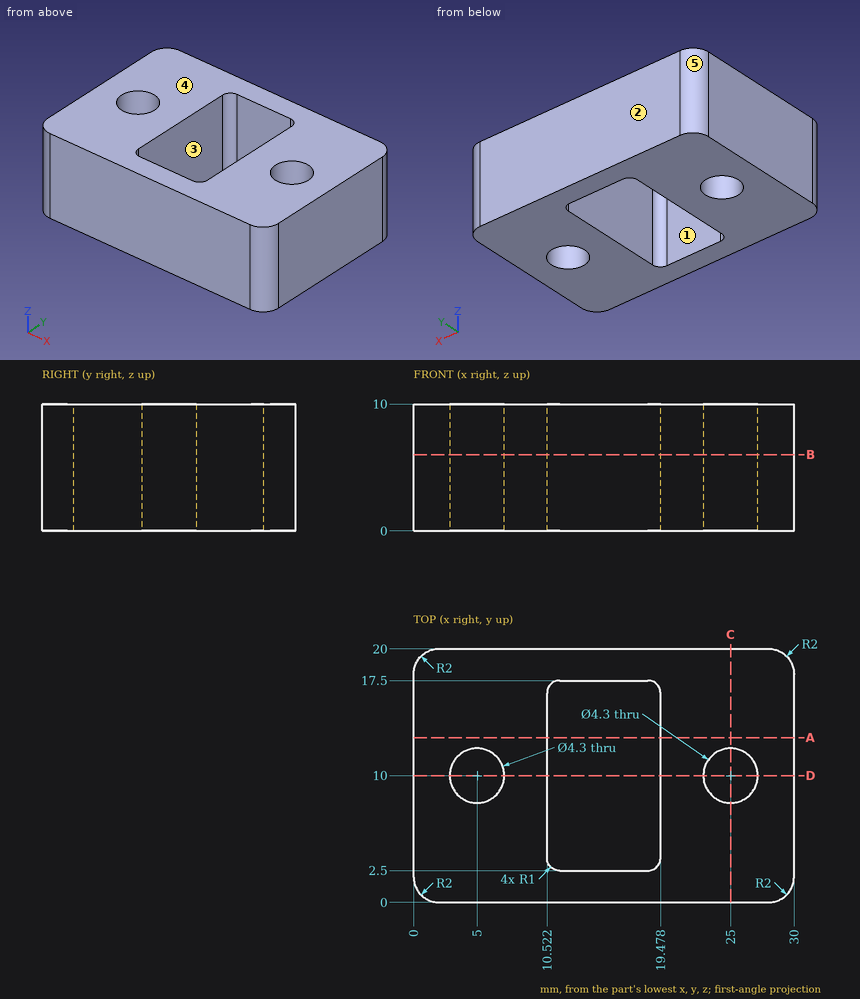
Part print with two shaded views. Sizes in mm from the minimum x, y, z corner. A direction names the side the tool comes from. Give positions to 0.01 mm unless a question says otherwise; leave off trailing zeros. Order: outer loops, then holes, each group sorted by start corner. A loop starts at its lowest first (then second) coordinate and runs counter-clockwise, first axis right, second up.
(1) Mould opens along Y. For the marked faces 3, 4 and 5 say: released by +Y, released by -Y, zero draft, split by the parting line, or undercut.
(2) Saw through at C-C, the plane x = 25. Give the cut face in (y, z), then the cut area to 3 significant figures.
(3) Saw through at A-A, the plane y = 13. Give the cut face in (x, z).
(4) Drill centre lines: L1, parallel to Y at x = 16.5, z = 4; L2, parallel to X at y = 14.25, z = 9.25; L3, parallel to Y at x = 25, z = 6.75. Where is each one in solid material? Low to high.
(5) Saw through at B-B, the plane z = 6. Give the cut face in (x, y).
(6) Tool access for the marked faces 1 and 2: list every direction of +Z, -Z, +X, -X, +Y, -Y with a clear straight run to the whole face (end or side of a thin tool).
(7) Saw through at D-D, the plane y = 10. Give the cut face in (x, z), then the cut area to 3 significant figures.
Results found:
1. face 3: undercut
1. face 4: zero draft
1. face 5: released by +Y
2. outline: (0, 0) - (7.85, 0) - (7.85, 10) - (0, 10) - close; (12.15, 0) - (20, 0) - (20, 10) - (12.15, 10) - close
2. area: 157 mm2
3. outline: (0, 0) - (10.52, 0) - (10.52, 10) - (0, 10) - close; (19.48, 0) - (30, 0) - (30, 10) - (19.48, 10) - close
4. L1: y = 0 to 2.5, 17.5 to 20
4. L2: x = 0 to 10.52, 19.48 to 30
4. L3: y = 0 to 7.85, 12.15 to 20
5. outline: (0, 2) arc R2 ccw to (2, 0) - (28, 0) arc R2 ccw to (30, 2) - (30, 18) arc R2 ccw to (28, 20) - (2, 20) arc R2 ccw to (0, 18) - close; hole circle Ø4.3 at (5, 10); hole (10.52, 3.5) arc R1 ccw to (11.52, 2.5) - (18.48, 2.5) arc R1 ccw to (19.48, 3.5) - (19.48, 16.5) arc R1 ccw to (18.48, 17.5) - (11.52, 17.5) arc R1 ccw to (10.52, 16.5) - close; hole circle Ø4.3 at (25, 10)
6. face 1: +Z, -Z
6. face 2: +Z, -Z, +X, -X, +Y
7. outline: (0, 0) - (2.85, 0) - (2.85, 10) - (0, 10) - close; (7.15, 0) - (10.52, 0) - (10.52, 10) - (7.15, 10) - close; (19.48, 0) - (22.85, 0) - (22.85, 10) - (19.48, 10) - close; (27.15, 0) - (30, 0) - (30, 10) - (27.15, 10) - close
7. area: 124 mm2
